Check sheet for the modelled part. Datum: model origin and axes. Units: mm. A direction names the side the tool comes from. Coordinates: 2 decimals unless noted, no trailing zeros. Loops run counter-clockwise (first coordinate to the right, second up) from the corner with the lowest first, then second, coordinate; pieces in that order, holes last.
Autodesk Inventor part; units mm, degrees
ref_plane "YZ Plane" through (0, 0, 0) normal (1, 0, 0) x (0, 1, 0)
ref_plane "XZ Plane" through (0, 0, 0) normal (0, 1, 0) x (-1, 0, 0)
ref_plane "XY Plane" through (0, 0, 0) normal (0, 0, 1) x (1, 0, 0)
sketch "Sketch1" plane through (0, 0, 0) normal (0, 0, 1) x (1, 0, 0)
  line L0 (-111.7609, 28.9288) -> (-11.7609, 28.9288)
  line L1 (-11.7609, 28.9288) -> (-11.7609, 18.9288)
  line L2 (-11.7609, 18.9288) -> (-111.7609, 18.9288)
  line L3 (-111.7609, 18.9288) -> (-111.7609, 28.9288)
  arc A0 (-111.7609, 28.9288) -> (-111.7609, 18.9288) centre (-111.7609, 23.9288) ccw
  arc A1 (-11.7609, 18.9288) -> (-11.7609, 28.9288) centre (-11.7609, 23.9288) ccw
  point P0 (0, 0)
  point P1 (-105.9495, 22.4367)
extrude "Extrusion1" add sketch "Sketch1" along normal blind 5
sketch "Sketch2" plane through (0, 0, 5) normal (0, 0, 1) x (1, 0, 0)
  circle A0 centre (-11.7633, 23.7843) radius 1.841
  circle A1 centre (-111.5799, 23.7843) radius 1.841
  point P0 (0, 0)
extrude "Extrusion2" cut sketch "Sketch2" against normal blind 5
sketch "Sketch3" plane through (0, 0, 5) normal (0, 0, 1) x (1, 0, 0)
  line L0 (-105.444, 25.5006) -> (-17.9751, 25.5006)
  line L1 (-17.9751, 25.5006) -> (-17.9751, 22.2171)
  line L2 (-17.9751, 22.2171) -> (-105.444, 22.2171)
  line L3 (-105.444, 22.2171) -> (-105.444, 25.5006)
  point P0 (0, 0)
extrude "Extrusion3" cut sketch "Sketch3" against normal blind 10
properties part number "Bracket"
1) Mould release check, pull along X, two halves, no side actions. Record for faces 1 (the flat face through (-105.444, 24, 3)), 2 (the flat face through (-61, 18.929, 2)), 3 (the cylindrical face through (-10.914, 22.151, 2.535)), 4 (the cylindrical face through (-116.76, 23.82, 2.46)): +X half, -X half, draft (parallel to the pull), parting line (faces both ways), or undercut.
Answer sheet:
face 1: undercut
face 2: draft
face 3: undercut
face 4: -X half
2) Section check C-C on y = 20. Enter the section's corners in (x, z).
Answer sheet:
outline: (-114.85, 0) - (-8.67, 0) - (-8.67, 5) - (-114.85, 5) - close
3) Section check D-D on y = 27.75. Enter the section's corners in (x, z).
Answer sheet:
outline: (-114.99, 0) - (-8.54, 0) - (-8.54, 5) - (-114.99, 5) - close
4) Set-up check for faces 5 (the flat face through (-61, 22.217, 3)), 6 (the cylindrical face through (-6.762, 24.039, 2.465)): record each of +Z, -Z, +X, -X, +Y, -Y from which the full face is reachable in a straight line by a thin tool's end or side.
Answer sheet:
face 5: +Z, -Z
face 6: +Z, -Z, +X
5) Scan lines: line 1 (X direction, y = 24, z = 0.6); line 2 (X direction, y = 23.5, z = 4.1); line 3 (Y direction, x = -32, z = 2.35). Record each from-to range of solid material in increasing order.
Answer sheet:
line 1: x = -116.76 to -113.41, -109.75 to -105.44, -17.98 to -13.59, -9.93 to -6.76
line 2: x = -116.74 to -113.4, -109.76 to -105.44, -17.98 to -13.58, -9.94 to -6.78
line 3: y = 18.93 to 22.22, 25.5 to 28.93
6) Section check A-A on x = -60. Enter the section's corners in (y, z).
Answer sheet:
outline: (18.93, 0) - (22.22, 0) - (22.22, 5) - (18.93, 5) - close; (25.5, 0) - (28.93, 0) - (28.93, 5) - (25.5, 5) - close
7) Depth check by flat-ended pin: pin 1 (1 mm diameter, centred on y = 21, z = 1.5, fed in from -X). Enter the tip coordinate at first touch or a pass-through.
Answer sheet:
pin 1: stops at x = -116.13
8) Section check B-B on z = 1.8. Enter the section's corners in (x, y), plus the area to 3 significant figures.
Answer sheet:
outline: (-111.76, 18.93) - (-11.76, 18.93) arc R5 ccw to (-11.76, 28.93) - (-111.76, 28.93) arc R5 ccw to start; hole circle Ø3.68 at (-111.58, 23.78); hole (-105.44, 22.22) - (-17.98, 22.22) - (-17.98, 25.5) - (-105.44, 25.5) - close; hole circle Ø3.68 at (-11.76, 23.78)
area: 770 mm2
